```python
from build123d import *

# Parameters (mm, degrees)
SKETCH_1_W          = 30
SKETCH_1_H          = 30
SKETCH_1_W_2        = 27
SKETCH_1_H_2        = 27
EXTRUDE_1_DEPTH     = 60
SKETCH_2_R          = 2.05
CUT_EXTRUDE_1_DEPTH = 69.738635424
SKETCH_3_R          = 2.05
CUT_EXTRUDE_2_DEPTH = 69.738635424
CUT_EXTRUDE_4_DEPTH = 69.738635424


with BuildPart() as part:
    # 草图1 → 凸台-拉伸1 (new body)
    with BuildSketch(Plane.XY):
        Rectangle(SKETCH_1_W, SKETCH_1_H)
        Rectangle(SKETCH_1_W_2, SKETCH_1_H_2, mode=Mode.SUBTRACT)
    extrude(amount=EXTRUDE_1_DEPTH)

    # 草图2 → 切除-拉伸1 (cut, through all)
    with BuildSketch(Plane(origin=(0, 15, 0), x_dir=(1, 0, 0), z_dir=(0, 1, 0))):
        with Locations(Location((-10, -7.5, 0), (0, 0, 270))):
            Circle(SKETCH_2_R)
        with Locations(Location((10, -7.5, 0), (0, 0, 270))):
            Circle(SKETCH_2_R)
        with Locations(Location((-10, -52.5, 0), (0, 0, 270))):
            Circle(SKETCH_2_R)
        with Locations(Location((10, -52.5, 0), (0, 0, 270))):
            Circle(SKETCH_2_R)
    extrude(amount=-CUT_EXTRUDE_1_DEPTH, mode=Mode.SUBTRACT)

    # 草图3 → 切除-拉伸2 (cut, through all)
    with BuildSketch(Plane(origin=(15, 0, 0), x_dir=(0, 0, -1), z_dir=(1, 0, 0))):
        with Locations(Location((-39, 10, 0), (0, 0, 90))):
            Circle(SKETCH_3_R)
        with Locations(Location((-39, -10, 0), (0, 0, 90))):
            Circle(SKETCH_3_R)
        with Locations(Location((-15, -10, 0), (0, 0, 90))):
            Circle(SKETCH_3_R)
        with Locations(Location((-15, 10, 0), (0, 0, 90))):
            Circle(SKETCH_3_R)
    extrude(amount=-CUT_EXTRUDE_2_DEPTH, mode=Mode.SUBTRACT)

    # 草图5 → 切除-拉伸4 (cut, through all)
    with BuildSketch(Plane(origin=(15, 0, 0), x_dir=(0, 0, -1), z_dir=(1, 0, 0))):
        Polygon((0, -15), (-11, 15), (0, 15), align=None)
    extrude(amount=-CUT_EXTRUDE_4_DEPTH, mode=Mode.SUBTRACT)


solid = part.part
```
Work out the finished part from the listing and answer in its coordinate system (mm). A direction names the side the tool comes from. Give positions to 0.01 mm unless a question says otherwise; leave off trailing zeros. Write each loop counter-clockwise with the first axis right and the second up, starting at its lowest first coordinate (ties: lowest second). Pieces come first, ordered by that corner, then holes.
(1) The part is cut by section A-A on x = 2. Write down the section's boundary in (y, z), plus the area to 4 significant figures.
Final values:
outline: (-15, 0) - (-13.5, 0.55) - (-13.5, 60) - (-15, 60) - close; (13.5, 10.45) - (15, 11) - (15, 60) - (13.5, 60) - close
area: 163.5 mm2
(2) The part is cut by section D-D on y = 10. Write down the section's boundary in (x, z), plus the area to 3 significant figures.
Final values:
outline: (-15, 9.17) - (-13.5, 9.17) - (-13.5, 12.95) - (-15, 12.95) - close; (-15, 17.05) - (-13.5, 17.05) - (-13.5, 36.95) - (-15, 36.95) - close; (-15, 41.05) - (-13.5, 41.05) - (-13.5, 60) - (-15, 60) - close; (13.5, 9.17) - (15, 9.17) - (15, 12.95) - (13.5, 12.95) - close; (13.5, 17.05) - (15, 17.05) - (15, 36.95) - (13.5, 36.95) - close; (13.5, 41.05) - (15, 41.05) - (15, 60) - (13.5, 60) - close
area: 128 mm2
(3) Which of the six approach directions +Z, -Z, +X, -X, +Y, -Y give full straight-line access (tool end or side, diameter ignored) to faces 1 (the cylindrical face through (-14.24, 7.95, 15.09)), 2 (the flat face through (0, 13.5, 35))?
Final values:
face 1: +X, -X
face 2: +Z, -Z
(4) Straight lines are drawn through the part: line 1 (X direction, y = -13, z = 57); line 2 (Z direction, x = 14.2, y = -10). For each, find the intervals that lie inside material, in ascending order.
Final values:
line 1: x = -15 to -13.5, 13.5 to 15
line 2: z = 1.83 to 12.95, 17.05 to 36.95, 41.05 to 60
(5) The part is cut by section C-C on z = 15. Write down the section's boundary in (x, y), plus the area to 3 significant figures.
Final values:
outline: (-15, -15) - (15, -15) - (15, -12.05) - (13.5, -12.05) - (13.5, -13.5) - (-13.5, -13.5) - (-13.5, -12.05) - (-15, -12.05) - close; (-15, -7.95) - (-13.5, -7.95) - (-13.5, 7.95) - (-15, 7.95) - close; (-15, 12.05) - (-13.5, 12.05) - (-13.5, 13.5) - (13.5, 13.5) - (13.5, 12.05) - (15, 12.05) - (15, 15) - (-15, 15) - close; (13.5, -7.95) - (15, -7.95) - (15, 7.95) - (13.5, 7.95) - close
area: 146 mm2
(6) Flat-ended cylindrical pins translate along their axes: pin 1 Ø1 at (x, y) = (-12, 9) entering from +Z; pin 2 Ø10 at (x, y) = (-9.5, -0.5) entering from -Z. Find the tip coordinate at first contact, or state that the pin passes through.
Final values:
pin 1: passes through
pin 2: stops at z = 4.22
(7) The mould has two halves that part along Z. Classify faces 3 (the cylindrical face through (14.26, -12.05, 15.09)), 4 (the flat face through (-14.374, -1.181, 5.067)), 5 (the flat face through (0, -15, 30)): pulls with the +Z half, pulls with the -Z half, needs draft (parallel to the pull), parting line crosses it, or undercut.
Final values:
face 3: undercut
face 4: pulls with the -Z half
face 5: needs draft
(8) The part is cut by section B-B on x = -10. Write down the section's boundary in (y, z).
Final values:
outline: (-15, 0) - (-13.5, 0.55) - (-13.5, 5.45) - (-15, 5.45) - close; (-15, 9.55) - (-13.5, 9.55) - (-13.5, 50.45) - (-15, 50.45) - close; (-15, 54.55) - (-13.5, 54.55) - (-13.5, 60) - (-15, 60) - close; (13.5, 10.45) - (15, 11) - (15, 50.45) - (13.5, 50.45) - close; (13.5, 54.55) - (15, 54.55) - (15, 60) - (13.5, 60) - close
